```python
from build123d import *

# Parameters (mm, degrees)
F1_DEPTH = 25


with BuildPart() as f1:
    # F0 (on Front) → F1 (new body)
    with BuildSketch(Plane.XZ):
        Polygon((-23.6734980222, 39.0396707756), (-32.0782363415, 38.9619767666), (-32.0782363415, 17.6561103577), (-23.6734980222, 17.6561103577), align=None)
        Polygon((-32.1401390579, 45.6584536185), (-32.0782363415, 38.9619767666), (-23.6734980222, 39.0396707756), (-12.5234980222, 39.0008237711), (-12.5234980222, 45.7367198607), (-23.6734980222, 45.7367198607), align=None)
        Polygon((-12.5234980222, 45.7367198607), (-12.5234980222, 39.0008237711), (-1.3734980222, 38.9619767666), align=None)
        Polygon((-1.3734980222, 38.9619767666), (-12.5234980222, 39.0008237711), (-12.5234980222, -21.1397777129), (-1.3734980222, -6.4730470867), align=None)
        Polygon((-12.5234980222, 45.7367198607), (-1.3734980222, 38.9619767666), (-1.3734980222, 45.7367198607), align=None)
        Polygon((-1.3734980222, -6.4730470867), (-12.5234980222, -21.1397777129), (-1.3734980222, -21.1397777129), align=None)
        Polygon((15.7792718965, 16.0897381949), (-1.3734980222, -6.4730470867), (-1.3734980222, -21.1397777129), (24.3684463203, 8.6735142395), align=None)
    extrude(amount=F1_DEPTH)


solid = f1.part
```
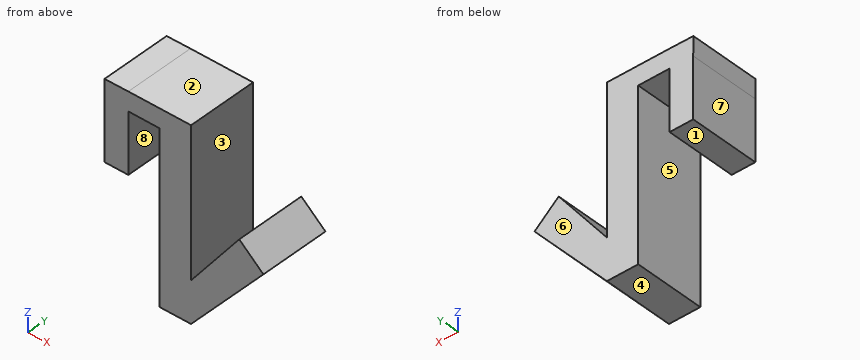
Geometry: final body of the model. Coordinates: model frame, mm. Face numbers are marked on the shaded views. A direction names the side the tool comes from. Round coordinates to 2 decimals unless told otherwise and drop trailing zeros. Order: outer loops, then holes, each group sorted by start corner. A loop starts at its lowest first (then second) coordinate and runs counter-clockwise, first axis right, second up. Notation, with made-up numbers: (-37.5, 71.5) -> (-17.5, 71.5) arc R22 cw to (-17.5, 84.5) -> close; hole circle Ø5 at (66, 49.25). An arc over 180 degrees is marked (long way). Use one line per item in the form item = value. Start each with the question number.
1. Draft query along X for the marked faces 6, 7 and 8. Return one class per face: pulls with the +X half, pulls with the -X half, needs draft (parallel to the pull), parting line crosses it, or undercut.
2. Reachability of the marked faces 1, 2, 3, 4 and 5 from +Z, -Z, +X, -X, +Y, -Y: full face, straight path, thin tool, end or side. Return the list, or none.
3. Cut plane A-A (z = 12). Return the cut outline in (x, y).
4. Cut plane D-D (x = 11.5). Return the cut outline in (y, z).
5. Cut plane C-C (z = 32). Return the cut outline in (x, y), then the cut area to 3 significant figures.
6. Cut plane B-B (y = -15.75). Return the cut outline in (x, z), then the cut area to 3 significant figures.
7. Pin query (flat end, axial travel): pin 1 Ø5 at (y, z) = (-14.5, 22.5) entering from -X; pin 2 Ø2 at (x, y) = (2, -16) entering from +Z; pin 3 Ø9 at (x, y) = (-26, -16.5) entering from -Z; pin 4 Ø5 at (x, z) = (-13, -1) entering from +Y. Return the tip coordinate at first contact, or that it passes through.
8. Line query: probe 1 along X at (y, z) = (-4.5, 25); probe 2 along Z at (x, y) = (-21, -3.5); probe 3 along X at (y, z) = (-20.75, 11). Output: solid intervals per line, ascending.
Solution:
q1.face_6 = needs draft
q1.face_7 = pulls with the -X half
q1.face_8 = undercut
q2.face_1 = -Z, -X, +Y, -Y
q2.face_2 = +Z, +X, -X, +Y, -Y
q2.face_3 = +Z, +Y, -Y
q2.face_4 = -Z, +X, -X, +Y, -Y
q2.face_5 = -Z, +Y, -Y
q3.outline = (-12.52, -25) -> (-1.37, -25) -> (-1.37, 0) -> (-12.52, 0) -> close; (12.67, -25) -> (20.52, -25) -> (20.52, 0) -> (12.67, 0) -> close
q4.outline = (-25, -6.23) -> (0, -6.23) -> (0, 10.46) -> (-25, 10.46) -> close
q5.outline = (-32.08, -25) -> (-23.67, -25) -> (-23.67, 0) -> (-32.08, 0) -> close; (-12.52, -25) -> (-1.37, -25) -> (-1.37, 0) -> (-12.52, 0) -> close
q5.area = 489 mm^2
q6.outline = (-32.14, 45.66) -> (-32.08, 38.96) -> (-32.08, 17.66) -> (-23.67, 17.66) -> (-23.67, 39.04) -> (-12.52, 39) -> (-12.52, -21.14) -> (-1.37, -21.14) -> (24.37, 8.67) -> (15.78, 16.09) -> (-1.37, -6.47) -> (-1.37, 45.74) -> (-23.67, 45.74) -> close
q6.area = 1,410 mm^2
q7.pin_1 = -32.08
q7.pin_2 = -0.72
q7.pin_3 = 17.66
q7.pin_4 = 0
q8.probe_1 = -32.08 to -23.67, -12.52 to -1.37
q8.probe_2 = 39.03 to 45.74
q8.probe_3 = -12.52 to -1.37, 11.91 to 21.67
